Work out the finished part from the listing and answer in its coordinate system (mm). A direction names the side the tool comes from. Give positions to 0.01 mm unless a question says otherwise; leave off trailing zeros. Loops run counter-clockwise (first coordinate to the right, second up) from the corner with the lowest first, then second, coordinate; pieces in that order, holes last. Notation, with made-up numbers: M 43,-23 L 94,-23 A20 ccw 94,-18 Z; hole C 4,37 d5. An arc over 180 degrees is marked long. Answer as a JSON object with one key per item and string values. Group by question number.
Autodesk Fusion 360 part; units mm, degrees
sketch "Schizzo1" plane through (0, 0, 0) normal (0, 0, 1) x (1, 0, 0)
  line L0 (0, 0) -> (-56.8, 0)
  line L1 (-56.8, 0) -> (-56.8, 16.7)
  line L2 (-56.8, 16.7) -> (0, 16.7)
  line L3 (0, 16.7) -> (0, 0)
  line L4 (0, 0) -> (0, 8.35)
  line L5 (0, 8.35) -> (-56.8, 8.35)
  line L6 (-56.8, 8.35) -> (-48.7, 8.35)
  line L7 (0, 8.35) -> (-8.1, 8.35)
  circle A0 centre (-48.7, 8.35) radius 1.5
  circle A1 centre (-8.1, 8.35) radius 1.5
  dimension "d1" = 56.8
  dimension "d2" = 16.7
  dimension "d3" = 8.1
  dimension "d4" = 8.1
  dimension "d5" = 3
  dimension "d6" = 3
extrude "Estrusione1" add sketch "Schizzo1" along normal blind 10 contours L5 L7 A1 | L5 L7 A1 | L5 L6 A0 | L5 L6 A0 makes body 1 at (-48.4395, 6.8728, 6.6667) makes body 2 at (-6.6075, 8.4994, 6.6667)
sketch "Schizzo2" plane through (0, 0, 0) normal (0, 0, 1) x (1, 0, 0)
  line L0 (0, 0) -> (-56.7, 0)
  line L1 (-56.7, 0) -> (-56.7, 16.7)
  line L2 (-56.7, 16.7) -> (0, 16.7)
  line L3 (0, 16.7) -> (0, 0)
  dimension "d9" = 56.7
  dimension "d10" = 16.7
extrude "Estrusione2" add sketch "Schizzo2" along normal blind 5 bodies 1 2
Item 1: For a pull along X with two mould halves and no side action, classify faces 3 (the flat face through (-29, 8, 0)), 4 (the flat face through (0, 8, 2)), 5 (the cylindrical face through (-8.295, 6.863, 7.465)) as pulls with the +X half, pulls with the -X half, needs draft (parallel to the pull), parting line crosses it, or undercut.
Item 2: A cutting plane is placed at D-D (y = 1.25). Determine the outline of the cut face in (x, z).
Item 3: Given pin 1 Ø4 at (x, z) = (-47.5, 7.5) entering from -Y; pin 2 Ø4 at (x, y) = (-23, 3) entering from +Z, each flat-ended and moving along its own axis, determine where each tip first touches the part or whether it passes through.
Item 4: A cutting plane is placed at C-C (y = 8.35). Determine the outline of the cut face in (x, z).
Item 5: A cutting plane is placed at A-A (x = -8.1). Determine the outline of the cut face in (y, z), and give its area (3 significant figures).
Item 6: A tool of negligible diameter and unlimited length cuts with its end or side. For faces 1 (the cylindrical face through (-47.27, 7.9, 7.46)), 2 (the flat face through (-28, 0, 2)), from which of +Z, -Z, +X, -X, +Y, -Y can it reach the whole face along a straight path? Write none if from no direction.
Item 7: A cutting plane is placed at B-B (z = 7). Determine the outline of the cut face in (x, y), and give its area (3 significant figures).
Item 8: Find the intervals of material crossed by probe 1 along Z at (x, y) = (-29, 15.5); probe 2 along X at (y, z) = (9, 8.5); probe 3 along Y at (x, z) = (-48, 8), in increasing order. Write a range as [from, to].
The answers:
{
 "1": {"face 3": "needs draft", "face 4": "pulls with the +X half", "face 5": "undercut"},
 "2": {"outline": "M -56.7,0 L 0,0 L 0,5 L -56.7,5 Z"},
 "3": {"pin 1": "stops at y = 6.85", "pin 2": "stops at z = 5"},
 "4": {"outline": "M -56.7,0 L 0,0 L 0,5 L -6.6,5 L -6.6,10 L -9.6,10 L -9.6,5 L -47.2,5 L -47.2,10 L -50.2,10 L -50.2,5 L -56.7,5 Z"},
 "5": {"outline": "M 0,0 L 16.7,0 L 16.7,5 L 9.85,5 L 9.85,10 L 6.85,10 L 6.85,5 L 0,5 Z", "area": "98.5 mm^2"},
 "6": {"face 1": "+Z", "face 2": "+Z, -Z, +X, -X, -Y"},
 "7": {"outline": "C -48.7,8.35 d3; C -8.1,8.35 d3", "area": "14.1 mm^2"},
 "8": {"probe 1": "z = [0, 5]", "probe 2": "x = [-50.05, -47.35], [-9.45, -6.75]", "probe 3": "y = [7.02, 9.68]"}
}
